Check sheet for the drawn part. Datum: minimum x, y, z corner. Units: mm. A direction names the side the tool comes from. Coordinates: 2 decimals unless noted, no trailing zeros. Loops run counter-clockwise (first coordinate to the right, second up) from the corner with the lowest first, then second, coordinate; pieces in that order, holes last.
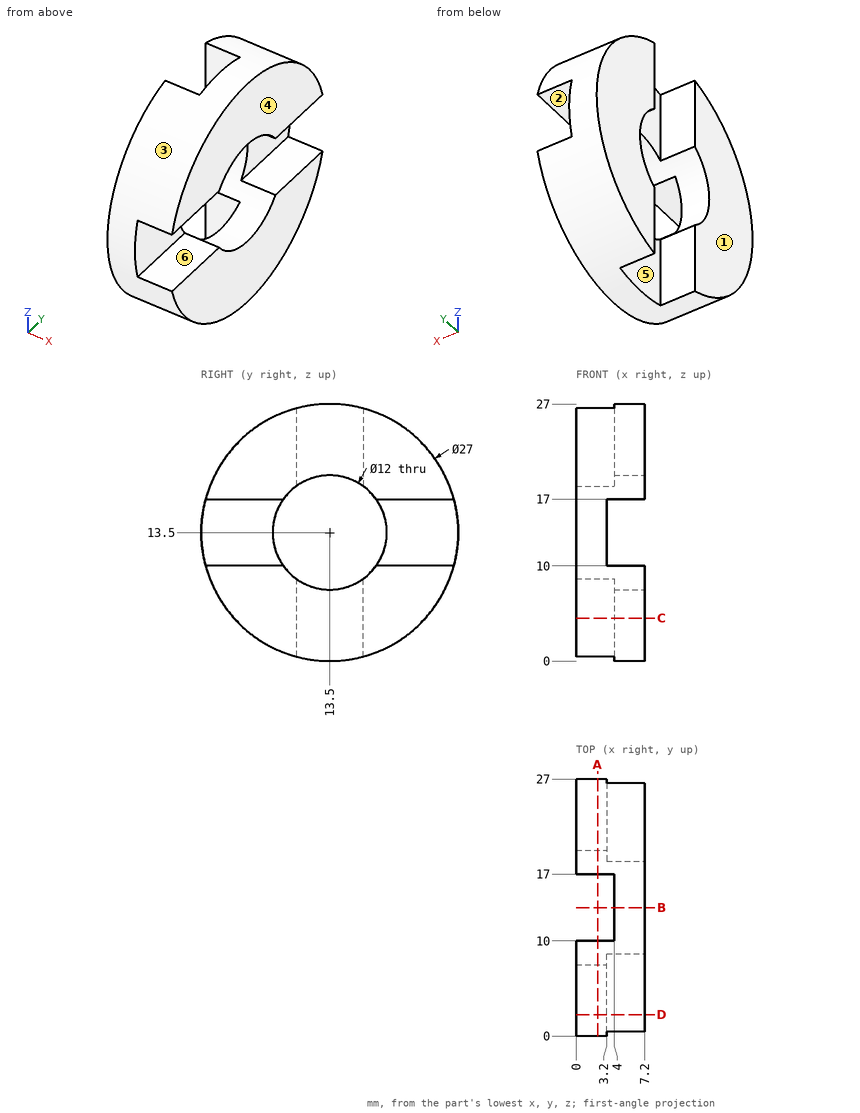
(1) Scan lines: L1, parallel to X at y = 3.5, z = 10.5; L2, parallel to X at y = 16.25, z = 6.5; L3, parallel to Y at x = 1.75, z = 22.25. Record each from-to range of solid material in increasing order.
Findings:
L1: x = 0 to 3.2
L2: x = 4 to 7.2
L3: y = 3.22 to 10, 17 to 23.78
(2) Access from +Z, -Z, +X, -X, +Y, -Y to the whole of each face (thin tool, end or side, straight path). Record for the marked faces 4, 5 and 6.
Findings:
face 4: +Z, -Z, +X, +Y, -Y
face 5: +Z, -Z, -X
face 6: +X, +Y, -Y
(3) Sectioned sample at B-B on y = 13.5. Record the cut outline in (x, z).
Findings:
outline: (4, 0) - (7.2, 0) - (7.2, 7.5) - (4, 7.5) - close; (4, 19.5) - (7.2, 19.5) - (7.2, 27) - (4, 27) - close
(4) Sectioned sample at D-D on y = 2.25. Record the cut outline in (x, z), and give its area (3 significant figures).
Findings:
outline: (0, 6.04) - (7.2, 6.04) - (7.2, 10) - (3.2, 10) - (3.2, 17) - (7.2, 17) - (7.2, 20.96) - (0, 20.96) - close
area: 79.5 mm2
(5) Draft check along Z on the marked faces 1, 2 and 3. Enter one of: +Z half, -Z half, draft (parallel to the pull), parting line (faces both ways), or undercut.
Findings:
face 1: draft
face 2: undercut
face 3: parting line
(6) Sectioned sample at A-A on x = 2.25. Record the cut outline in (y, z).
Findings:
outline: (10, 0.46) - (10, 8.63) arc R6 cw to (10, 18.37) - (10, 26.54) arc R13.5 ccw to start; (17, 0.46) arc R13.5 ccw to (17, 26.54) - (17, 18.37) arc R6 cw to (17, 8.63) - close
(7) Sectioned sample at C-C on z = 4.5. Record the cut outline in (x, y).
Findings:
outline: (0, 3.44) - (7.2, 3.44) - (7.2, 23.56) - (0, 23.56) - (0, 17) - (4, 17) - (4, 10) - (0, 10) - close
(8) Gauge pin test, flat ends, axial feed: pin 1 Ø3 at (x, y) = (5, 20.5) entering from -Z; pin 2 Ø2 at (x, z) = (2, 22.5) entering from -Y; pin 3 Ø1.2 at (x, z) = (1, 2.5) entering from -Y. Record the tip position at first contact, or that the pin passes through.
Findings:
pin 1: stops at z = 1.17
pin 2: stops at y = 2.63
pin 3: stops at y = 4.89
